Part print with two shaded views. Sizes in mm from the minimum x, y, z corner. A direction names the side the tool comes from. Round coordinates to 2 decimals unless told otherwise and drop trailing zeros. Order: outer loops, then holes, each group sorted by start corner. A loop starts at its lowest first (then second) coordinate and runs counter-clockwise, first axis right, second up. Notation, with made-up numbers: (54, -5.75) - (99, -5.75) arc R23 ccw to (99, 26.25) - close; hole circle Ø9 at (-11, 35). An arc over 180 degrees is marked (long way). Use one line per item in the form item = value.
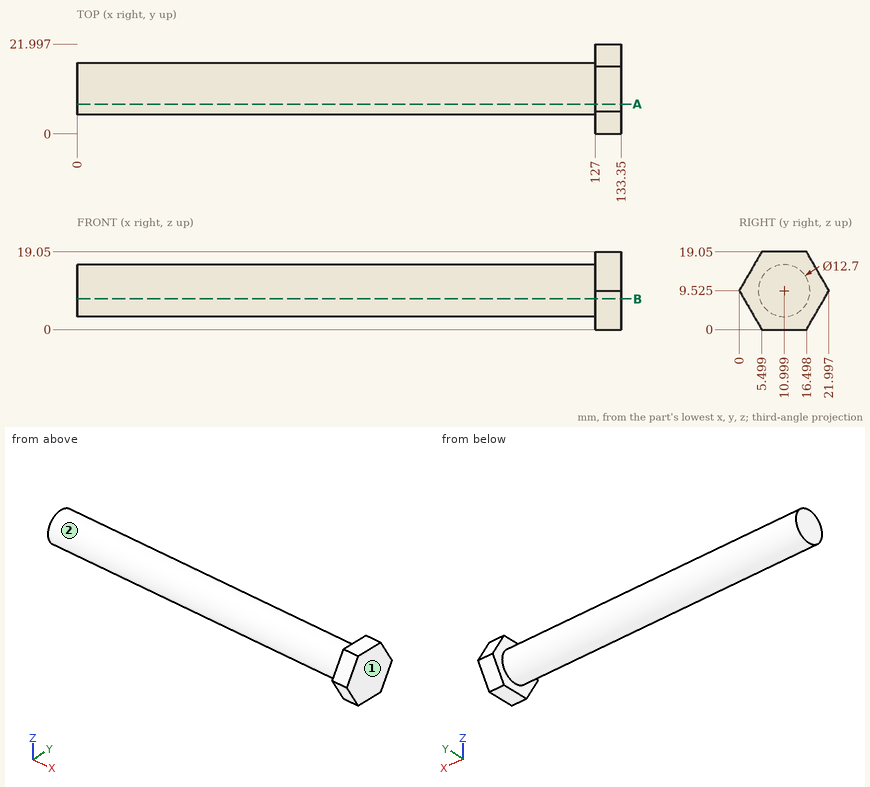
(1) Tool access for the marked faces 1 and 2: list every direction of +Z, -Z, +X, -X, +Y, -Y with a clear straight run to the whole face (end or side of a thin tool).
Report:
face_1 = +Z, -Z, +X, +Y, -Y
face_2 = -X
(2) Slice it at B-B on z = 7.5. Give the cut face in (x, y).
Report:
outline = (0, 4.98) - (127, 4.98) - (127, 1.17) - (133.35, 1.17) - (133.35, 20.83) - (127, 20.83) - (127, 17.02) - (0, 17.02) - close
(3) Probe probe 1 along X at (y, z) = (18.75, 5.5); probe 2 along Z at (x, y) = (55, 11.5) (1 decimal); probe 3 along Y at (x, z) = (67, 12.75). List the from-to ranges inside material, lowest first. Write a range as [from, to].
Report:
probe_1 = [127, 133.35]
probe_2 = [3.2, 15.9]
probe_3 = [5.53, 16.47]
(4) Slice it at A-A on y = 7.25. Give the cut face in (x, z).
Report:
outline = (0, 4.4) - (127, 4.4) - (127, 0) - (133.35, 0) - (133.35, 19.05) - (127, 19.05) - (127, 14.65) - (0, 14.65) - close
(5) Pin check, flat tips, straight feed: pin 1 (8 mm diameter, centred on x = 104.5, z = 15.5, fed in from +Y); pin 2 (4 mm diameter, centred on y = 7, z = 13, fed in from -X); pin 3 (6 mm diameter, centred on x = 87, z = 3, fed in from +Y); pin 4 (10 mm diameter, centred on x = 100, z = 11.5, fed in from +Y). Stop position of each tip, or through.
Report:
pin_1 = 17.03
pin_2 = 0
pin_3 = 16.28
pin_4 = 17.35
